Autodesk Inventor part; units mm, degrees
ref_plane "Work Plane2" through (0, 0, 0) normal (-1, 0, 0) x (0, 0, 1)
ref_plane "Work Plane4" through (-2.54, 0, 0) normal (-1, 0, 0) x (0, 0, 1)
ref_plane "Work Plane5" through (3.81, 0, 0) normal (1, 0, 0) x (0, 0, -1)
sketch "Sketch1" plane through (0, 0, 0) normal (1, 0, 0) x (0, 1, 0)
  circle A0 centre (0, 0) radius 3.937
  circle A1 centre (0, 0) radius 7.747
  dimension "d0" = 7.874
  dimension "d1" = 3.81
ref_plane "Work Plane2" through (0, 0, 0) normal (-1, 0, 0) x (0, 0, 1)
sketch "Sketch2" plane through (0, 0, 0) normal (-1, 0, 0) x (0, 0, 1)
  circle A0 centre (0, 0) radius 7.7384
  circle A1 centre (0, 0) radius 7.747
ref_plane "Work Plane4" through (-2.54, 0, 0) normal (-1, 0, 0) x (0, 0, 1)
sketch "Sketch3" plane through (-2.54, 0, 0) normal (-1, 0, 0) x (0, 0, 1)
  line L0 (19.05, 48.5955) -> (-19.05, 48.5955)
  circle A0 centre (0, 0) radius 7.747
  line L1 (7.747, 0) -> (19.05, 48.5955)
  line L2 (-7.747, 0) -> (-19.05, 48.5955)
  arc A1 (7.747, 0) -> (-7.747, 0) centre (0, 0) ccw
  line L3 (-14.2521, 44.7855) -> (14.2521, 44.7855)
  line L4 (14.2521, 44.7855) -> (6.1161, 9.806)
  arc A2 (6.1161, 9.806) -> (-6.1161, 9.806) centre (0, 0) ccw
  line L5 (-6.1161, 9.806) -> (-14.2521, 44.7855)
  dimension "d6" = 38.1
  dimension "d7" = 19.05
  dimension "d8" = 3.81
ref_plane "Work Plane5" through (3.81, 0, 0) normal (1, 0, 0) x (0, 0, -1)
sketch "Sketch4" plane through (3.81, 0, 0) normal (1, 0, 0) x (0, 0, -1)
  line L0 (14.2521, 44.7855) -> (6.1161, 9.806)
  line L1 (14.2521, 44.7855) -> (6.1161, 9.806)
  arc A0 (6.1161, 9.806) -> (-6.1161, 9.806) centre (0, 0) ccw
  line L2 (-6.1161, 9.806) -> (-14.2521, 44.7855)
  line L3 (-14.2521, 44.7855) -> (14.2521, 44.7855)
  line L4 (19.05, 48.5955) -> (-19.05, 48.5955)
  line L5 (-19.05, 48.5955) -> (-7.747, 0)
  line L6 (7.747, 0) -> (19.05, 48.5955)
  line L7 (-14.2521, 44.7855) -> (14.2521, 44.7855)
  line L8 (14.2521, 44.7855) -> (18.1638, 44.7855)
  line L9 (14.2521, 44.7855) -> (-14.2521, 44.7855)
  line L10 (-14.2521, 44.7855) -> (-18.1638, 44.7855)
  line L11 (-19.05, 48.5955) -> (-7.747, 0)
  line L12 (-19.05, 48.5955) -> (-18.1638, 44.7855)
  line L13 (18.1638, 44.7855) -> (19.05, 48.5955)
  line L14 (-19.05, 48.5955) -> (19.05, 48.5955)
  line L15 (19.05, 48.5955) -> (-19.05, 48.5955)
  line L16 (18.1638, 44.7855) -> (-18.1638, 44.7855)
  arc A1 (7.747, 0) -> (-7.747, 0) centre (0, 0) ccw
extrude "Extrusion4" add sketch "Sketch4" along normal blind 20.6375 contours L3 L10 L5 L4 L6 L8
ref_plane "Work Plane7" through (-2.54, 44.7855, -14.2521) normal (0, -1, 0) x (1, 0, 0)
ref_plane "Work Plane6" through (-2.54, 44.7855, -14.2521) normal (0, -1, 0) x (1, 0, 0)
sketch "Sketch6" plane through (-2.54, 44.7855, -14.2521) normal (0, -1, 0) x (1, 0, 0)
  line L0 (6.35, 32.4159) -> (26.9875, 32.4159)
  line L1 (13.4874, 32.4159) -> (13.4874, 26.0989)
  line L2 (26.9875, 32.4159) -> (26.9875, -3.9117)
  point P0 (2.54, 14.2521)
  dimension "d20" = 13.5001
ref_plane "Work Plane1" through (10.9347, 0, 0) normal (1, 0, 0) x (0, 0, -1)
ref_plane "Work Plane3" through (0, 0, 0) normal (1, 0, 0) x (0, 0, -1)
sketch "Sketch10" plane through (0, 0, 0) normal (1, 0, 0) x (0, 0, -1)
  circle A0 centre (0, 0) radius 1.4542
extrude "Extrusion7" cut sketch "Sketch10" against normal blind 22.225
sketch "Sketch12" plane through (3.81, 0, 0) normal (-1, 0, 0) x (0, 0, 1)
  line L0 (18.1638, 44.7855) -> (-18.1638, 44.7855)
  line L1 (19.05, 48.5955) -> (18.1638, 44.7855)
  line L2 (-19.05, 48.5955) -> (19.05, 48.5955)
  line L3 (-19.05, 48.5955) -> (19.05, 48.5955)
  line L4 (18.1638, 44.7855) -> (-18.1638, 44.7855)
  line L5 (-19.05, 48.5955) -> (19.05, 48.5955)
  line L6 (-18.1638, 44.7855) -> (-19.05, 48.5955)
  line L7 (18.1638, 44.7855) -> (-18.1638, 44.7855)
  line L8 (-19.05, 48.5955) -> (19.05, 48.5955)
  line L9 (19.05, 48.5955) -> (-19.05, 48.5955)
  line L10 (-9.4207, 44.7855) -> (-18.1638, 44.7855)
  line L11 (-19.05, 48.5955) -> (-18.1638, 44.7855)
  line L12 (18.1638, 44.7855) -> (-18.1638, 44.7855)
  line L13 (-18.1638, 44.7855) -> (18.1638, 44.7855)
  line L14 (18.1638, 44.7855) -> (19.05, 48.5955)
  line L15 (19.05, 48.5955) -> (18.1638, 44.7855)
  line L16 (19.05, 48.5955) -> (18.1638, 44.7855)
  line L17 (-18.1638, 44.7855) -> (-19.05, 48.5955)
  line L18 (-18.1638, 44.7855) -> (-19.05, 48.5955)
  point P0 (0, 0)
  point P1 (9.4207, 48.5955)
  point P2 (9.4207, 44.7855)
  point P3 (6.3245, 44.7855)
  point P4 (6.3245, 48.5955)
  point P5 (-6.3245, 48.5955)
  point P6 (-6.3245, 44.7855)
  point P7 (-9.4207, 48.5955)
extrude "Extrusion8" add sketch "Sketch12" along normal blind 6.35
sketch "Sketch13" plane through (24.4475, 44.7855, -18.1638) normal (0, -1, 0) x (1, 0, 0)
  line L0 (-26.9875, 0) -> (-26.9875, 36.3276)
  line L1 (0, 36.3276) -> (0, 0)
  line L2 (-26.9875, 36.3276) -> (0, 36.3276)
  line L3 (-26.9875, -0.8862) -> (0, -0.8862)
  line L4 (0, 37.2138) -> (-26.9875, 37.2138)
  point P0 (-24.4475, 18.1638)
  point P1 (-21.7476, 26.0364)
  point P2 (-21.7476, 10.2912)
  dimension "d35" = 21.7476
  dimension "d36" = 21.7476
  dimension "d38" = 11.1774
  dimension "d39" = 11.1774
ref_plane "Work Plane8" through (10.9537, 0, 0) normal (1, 0, 0) x (0, 0, -1)
hole "Hole2" at (2.6999, 44.7855, -7.8726) at (2.6999, 44.7855, 7.8726) direction (0, 1, 0) diameter 3.81 end through all
mirror "Mirror2" about plane through (10.9537, 0, 0) normal (1, 0, 0) of "Hole2"
sketch "Sketch14" plane through (24.4475, 44.7855, -18.1638) normal (0, -1, 0) x (1, 0, 0)
  line L0 (-25.5905, 0.7648) -> (-22.5425, 0.7648)
  line L1 (-22.5425, 0.7648) -> (-22.5425, 3.8128)
  line L2 (-22.5425, 3.8128) -> (-25.5905, 3.8128)
  line L3 (-25.5905, 3.8128) -> (-25.5905, 0.7648)
  line L4 (-26.9875, -0.8862) -> (0, -0.8862)
  line L5 (-26.9875, 0) -> (-26.9875, 36.3276)
  line L6 (-25.5905, 32.6418) -> (-22.6695, 32.6418)
  line L7 (-22.6695, 32.6418) -> (-22.6695, 35.5628)
  line L8 (-22.6695, 35.5628) -> (-25.5905, 35.5628)
  line L9 (-25.5905, 35.5628) -> (-25.5905, 32.6418)
  line L10 (0, 37.2138) -> (-26.9875, 37.2138)
  point P0 (-24.4475, 18.1638)
  dimension "d47" = 3.048
  dimension "d48" = 3.048
  dimension "d49" = 1.651
  dimension "d50" = 1.397
  dimension "d51" = 2.921
  dimension "d52" = 2.921
  dimension "d53" = 1.651
  dimension "d54" = 1.397
extrude "Extrusion9" cut sketch "Sketch14" against normal blind 1.905
properties part number "BottomHolderThrustMotorHousing"
Geometry check sheet. Reference: the model listing, model coordinates, mm. A direction names the side the tool comes from. Give positions to 0.01 mm unless a question says otherwise; leave off trailing zeros. Loops run counter-clockwise (first coordinate to the right, second up) from the corner with the lowest first, then second, coordinate; pieces in that order, holes last. Notation, with made-up numbers: M 53,30.25 L 81,30.25 A7 cw 81,35.25 Z; hole C 76.5,12.5 d6. An arc over 180 degrees is marked long. Write each question's results on one line, items separated by ' | '.
1) Section check C-C, the plane y = 47.7. Record the boundary of the cut face in (x, z) (1 decimal), plus the area to 3 significant figures.
Answers follow:
outline: M -2.5,-18.8 L 24.4,-18.8 L 24.4,18.8 L -2.5,18.8 Z; hole C 2.7,-7.9 d3.8; hole C 2.7,7.9 d3.8; hole C 19.2,-7.9 d3.8; hole C 19.2,7.9 d3.8 | area: 971 mm2
2) Section check B-B, the plane z = -8.5. Record the boundary of the cut face in (x, y), plus the area to 3 significant figures.
Answers follow:
outline: M -2.54,44.79 L 0.9,44.79 L 0.9,48.6 L -2.54,48.6 Z; M 4.5,44.79 L 17.41,44.79 L 17.41,48.6 L 4.5,48.6 Z; M 21.01,44.79 L 24.45,44.79 L 24.45,48.6 L 21.01,48.6 Z | area: 75.4 mm2
3) Section check D-D, the plane z = 15. Record the boundary of the cut face in (x, y), plus the area to 3 significant figures.
Answers follow:
outline: M -2.54,44.79 L -1.14,44.79 L -1.14,46.69 L 1.78,46.69 L 1.78,44.79 L 24.45,44.79 L 24.45,48.6 L -2.54,48.6 Z | area: 97.3 mm2
4) Gauge pin test, flat ends, axial feed: pin 1 (1.5 mm diameter, centred on x = 0.5, z = 16, fed in from -Y); pin 2 (2 mm diameter, centred on x = 0.5, y = 46, fed in from +Z); pin 3 (1 mm diameter, centred on x = 0, y = 46, fed in from +Z); pin 4 (3 mm diameter, centred on x = 19.21, z = -7.87, fed in from -Y). Record the tip position at first contact, or that the pin passes through.
Answers follow:
pin 1: y = 46.69 | pin 2: z = 18.68 | pin 3: z = 18.56 | pin 4: through
5) Section check A-A, the plane y = 45.65. Record the boundary of the cut face in (x, z) (1 decimal), plus the area to 3 significant figures.
Answers follow:
outline: M -2.5,-18.4 L 24.4,-18.4 L 24.4,18.4 L -2.5,18.4 Z; hole M -1.1,-17.4 L 1.9,-17.4 L 1.9,-14.4 L -1.1,-14.4 Z; hole M -1.1,14.5 L 1.8,14.5 L 1.8,17.4 L -1.1,17.4 Z; hole C 2.7,-7.9 d3.8; hole C 2.7,7.9 d3.8; hole C 19.2,-7.9 d3.8; hole C 19.2,7.9 d3.8 | area: 928 mm2
6) Tool access check on faces 1 (the face through (0, 46, -14.351)), 2 (the face through (4.56, 46.72, 8.29)). Record the directions out of +Z, -Z, +X, -X, +Y, -Y that give a thin tool (end or side, any length) a straight path to the whole face; none if there is none.
Answers follow:
face 1: -Y | face 2: +Y, -Y
7) Thickness scan on line 1 (Z direction, x = 18.25, y = 46.1); line 2 (X direction, y = 45.5, z = 7); line 3 (Z direction, x = 18, y = 45.35). Record the ranges inside material, lowest first.
Answers follow:
line 1: -18.47 to -9.52, -6.23 to 6.23, 9.52 to 18.47 | line 2: -2.54 to 1.01, 4.39 to 17.51, 20.9 to 24.45 | line 3: -18.3 to -9.35, -6.4 to 6.4, 9.35 to 18.3
8) Release check for a two-part mould opening along Z. For faces 3 (the face through (11, 48.596, 0)), 4 (the face through (1.905, 46, -16)) record: +Z half, -Z half, draft (parallel to the pull), parting line (faces both ways), or undercut.
Answers follow:
face 3: draft | face 4: undercut
